Autodesk Inventor part; units mm, degrees
ref_plane "YZ Plane" through (0, 0, 0) normal (1, 0, 0) x (0, 1, 0)
ref_plane "XZ Plane" through (0, 0, 0) normal (0, 1, 0) x (-1, 0, 0)
ref_plane "XY Plane" through (0, 0, 0) normal (0, 0, 1) x (1, 0, 0)
sketch "Sketch1" plane through (0, 0, 0) normal (0, 0, 1) x (1, 0, 0)
  line L0 (0, 0) -> (-20, 0)
  line L1 (-20, 0) -> (-20, 55.5)
  line L2 (-20, 55.5) -> (0, 55.5)
  line L3 (0, 55.5) -> (0, 0)
  line L4 (-10, 0) -> (-10, 55.5) construction
  circle A0 centre (-10, 37.75) radius 2.6
  circle A1 centre (-10, 17.75) radius 2.6
  dimension "d0" = 20
  dimension "d1" = 55.5
  dimension "d2" = 5.2
  dimension "d3" = 5.2
  dimension "d4" = 17.75
  dimension "d5" = 17.75
extrude "Extrusion1" add sketch "Sketch1" along normal blind 5
sketch "Sketch2" plane through (0, 0, 0) normal (1, 0, 0) x (0, 0, -1)
  line L0 (0, 55.5) -> (-5, 55.5)
  line L1 (0, 55.5) -> (-24, 55.5)
  line L2 (-24, 55.5) -> (-24, 52)
  line L3 (-24, 52) -> (0, 52)
  line L4 (0, 52) -> (0, 55.5)
  line L5 (0, 0) -> (-5, 0)
  line L6 (0, 0) -> (-24, 0)
  line L7 (-24, 0) -> (-24, 3.5)
  line L8 (-24, 3.5) -> (0, 3.5)
  line L9 (0, 3.5) -> (0, 0)
  dimension "d8" = 24
  dimension "d9" = 3.5
  dimension "d10" = 24
  dimension "d11" = 3.5
extrude "Extrusion2" add sketch "Sketch2" along normal blind 26
fillet "Fillet1" radius 12 4 edges at (26, 53.75, 0) (26, 53.75, 24) (26, 1.75, 0) (26, 1.75, 24)
sketch "Sketch3" plane through (-20, 55.5, 5) normal (0, 1, 0) x (1, 0, 0)
  arc A0 (34, -19) -> (34, 5) centre (34, -7) ccw
  circle A1 centre (34, -7) radius 2.75
  point P0 (20, 5)
  dimension "d15" = 5.5
extrude "Extrusion3" cut sketch "Sketch3" against normal through all
chamfer "Chamfer1" distance 20 distance2 19 1 edges at (0, 53.75, 5) measured on face at (-17.5081, 30.8759, 5)
chamfer "Chamfer2" distance 20 distance2 19 1 edges at (0, 1.75, 5) measured on face at (-17.508, 23.4574, 5)
equation "\"d3\" = d2"
equation "\"d5\" = d4"
properties part number "Y Axis Drag Chain Mount Stationary"
Read the model definition and answer for the solid it produces. Units are mm, in the model's axes. A direction names the side the tool comes from. Coordinates: 2 decimals unless noted, no trailing zeros. Loops run counter-clockwise (first coordinate to the right, second up) from the corner with the lowest first, then second, coordinate; pieces in that order, holes last. Notation, with made-up numbers: (-28.75, -39.75) - (17.25, -39.75) arc R32 ccw to (17.25, -12.75) - close; hole circle Ø9 at (5.25, 53.5). An arc over 180 degrees is marked (long way). Answer in a Markdown table with one row per item.
1. Find section A-A, the plane y = 17.75. Write down the section's boundary in (x, z), then the cut area to 3 significant figures.
Conclusion:
| item | result |
|---|---|
| outline | (-20, 0) - (-12.6, 0) - (-12.6, 5) - (-20, 5) - close; (-7.4, 0) - (0, 0) - (0, 5) - (-7.4, 5) - close |
| area | 74.0 mm² |
2. Find section C-C, the plane z = 10.5. Write down the section's boundary in (x, y), then the cut area to 3 significant figures.
Conclusion:
| item | result |
|---|---|
| outline | (-14.21, 0) - (11.7, 0) - (11.7, 3.5) - (-14.21, 3.5) - close; (-14.21, 52) - (11.7, 52) - (11.7, 55.5) - (-14.21, 55.5) - close; (16.3, 0) - (25.91, 0) - (25.91, 3.5) - (16.3, 3.5) - close; (16.3, 52) - (25.91, 52) - (25.91, 55.5) - (16.3, 55.5) - close |
| area | 249 mm² |
3. Given pin 1 (1.5 mm diameter, centred on y = 26.5, z = 1.5, fed in from +X); pin 2 (10 mm diameter, centred on x = -10.5, y = 26.5, fed in from +Z); pin 3 (9 mm diameter, centred on x = 14, z = 12, fed in from -Y), each flat-ended and moving along its own axis, determine where each tip first touches the part or whether it passes through.
Conclusion:
| item | result |
|---|---|
| pin 1 | stops at x = 0 |
| pin 2 | stops at z = 5 |
| pin 3 | stops at y = 0 |
4. Which of the six approach directions +Z, -Z, +X, -X, +Y, -Y give full straight-line access (tool end or side, diameter ignored) to faces 4 (the face through (0, 28, 2)), 5 (the face through (8, 3.5, 12)), 6 (the face through (-7.6, 18.75, 2.46))?
Conclusion:
| item | result |
|---|---|
| face 4 | +Z, -Z, +X |
| face 5 | +Z, +X |
| face 6 | +Z, -Z |
5. Find section B-B, the plane x = -10. Write down the section's boundary in (y, z).
Conclusion:
| item | result |
|---|---|
| outline | (0, 0) - (15.15, 0) - (15.15, 5) - (3.5, 5) - (3.5, 14.5) - (0, 14.5) - close; (20.35, 0) - (35.15, 0) - (35.15, 5) - (20.35, 5) - close; (40.35, 0) - (55.5, 0) - (55.5, 14.5) - (52, 14.5) - (52, 5) - (40.35, 5) - close |
6. Determine the mould class of faces 1 (the face through (22.39, 1.73, 3.42)), 2 (the face through (-9.86, 53.77, 14.63)), 3 (the face through (11.973, 53.774, 10.141)) for opening direction X: +X half, -X half, draft (parallel to the pull), parting line (faces both ways), or undercut.
Conclusion:
| item | result |
|---|---|
| face 1 | +X half |
| face 2 | -X half |
| face 3 | undercut |
7. Find section D-D, the plane z = 16.5. Write down the section's boundary in (x, y).
Conclusion:
| item | result |
|---|---|
| outline | (-7.89, 0) - (25.12, 0) - (25.12, 3.5) - (-7.89, 3.5) - close; (-7.89, 52) - (25.12, 52) - (25.12, 55.5) - (-7.89, 55.5) - close |
8. Straight lines are drawn through the part: line 1 (Y direction, x = -10, z = 2.8); line 2 (Z direction, x = 14, y = 2); line 3 (Y direction, x = 17, z = 21.25). For each, find the intervals that lie inside material, in ascending order.
Conclusion:
| item | result |
|---|---|
| line 1 | y = 0 to 15.15, 20.35 to 35.15, 40.35 to 55.5 |
| line 2 | z = 0 to 9.25, 14.75 to 24 |
| line 3 | y = 0 to 3.5, 52 to 55.5 |
